Autodesk Inventor part; units mm, degrees
ref_plane "YZ Plane" through (0, 0, 0) normal (1, 0, 0) x (0, 1, 0)
ref_plane "XZ Plane" through (0, 0, 0) normal (0, 1, 0) x (-1, 0, 0)
ref_plane "XY Plane" through (0, 0, 0) normal (0, 0, 1) x (1, 0, 0)
sketch "Sketch1" plane through (0, 0, 0) normal (0, 1, 0) x (-1, 0, 0)
  circle A0 centre (0, 0) radius 73.025
  circle A1 centre (0, 0) radius 85.725
  line L0 (0, 0) -> (101.6, 0) construction
  line L1 (101.6, 0) -> (85.679, -2.8073)
  arc A2 (72.3305, -46.0117) -> (101.6, 0) centre (50.8, 0) ccw
  line L2 (-50.8, 87.9882) -> (-40.4083, 75.6039)
  arc A3 (3.6821, 85.6459) -> (-50.8, 87.9882) centre (-25.4, 43.9941) ccw
  line L3 (-50.8, -87.9882) -> (-45.2707, -72.7966)
  arc A4 (-76.0126, -39.6342) -> (-50.8, -87.9882) centre (-25.4, -43.9941) ccw
  arc A5 (78.2836, -34.935) -> (94.5805, -7.6857) centre (50.8, 0) ccw
  line L4 (94.5805, -7.6857) -> (85.215, -9.3371)
  line L5 (-40.6343, 85.752) -> (-34.5213, 78.4669)
  arc A6 (-8.8872, 85.2631) -> (-40.6343, 85.752) centre (-25.4, 43.9941) ccw
  line L6 (-53.9463, -78.0663) -> (-50.6936, -69.1298)
  arc A7 (-69.3964, -50.3281) -> (-53.9463, -78.0663) centre (-25.4, -43.9941) ccw
  point P0 (85.725, 0)
  point P1 (-42.8625, 74.24)
  point P2 (-42.8625, -74.24)
  point P3 (-8.8872, 85.2631)
  dimension "Ring_ID" = 146.05
  dimension "RingWD" = 12.7
  dimension "ToothDepth" = 15.875
  dimension "d4" = 10
  dimension "d5" = 50.8
  dimension "d8" = 360
  dimension "d13" = 6.35
  dimension "d14" = 6.35
  dimension "d17" = 360
extrude "Extrusion1" add sketch "Sketch1" along normal blind 9.525 contours A1 | A1 A6 L5 L2 A3 | L1 A2 A1 A5 L4 | A1 A7 L6 L3 A4
fillet "Fillet1" radius 3.175 6 edges at (40.4083, 4.7625, 75.6039) (-3.6821, 4.7625, 85.6459) (76.0126, 4.7625, -39.6342) (45.2707, 4.7625, -72.7966) (-85.679, 4.7625, -2.8073) (-72.3305, 4.7625, -46.0117)
fillet "Fillet2" radius 3.175 9 edges at (53.9463, 4.7625, -78.0663) (50.6936, 4.7625, -69.1298) (69.3964, 4.7625, -50.3281) (-94.5805, 4.7625, -7.6857) (-85.215, 4.7625, -9.3371) (-78.2836, 4.7625, -34.935) (40.6343, 4.7625, 85.752) (34.5213, 4.7625, 78.4669) (8.8872, 4.7625, 85.2631)
properties part number "Blade V2" material "Stainless Steel"
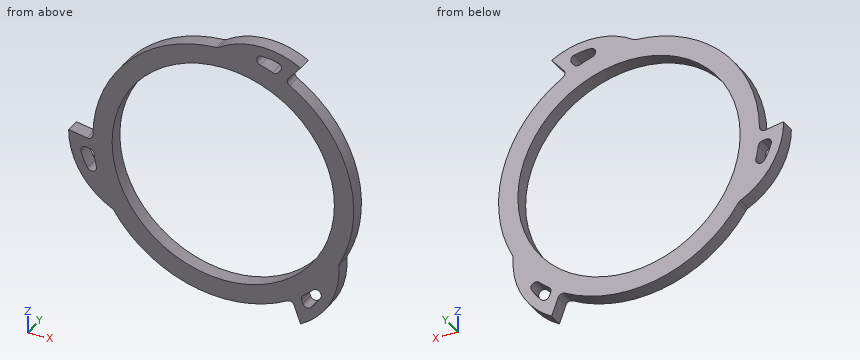
For this review, take the finished solid that the model builds, in its own axes (mm). Round coordinates to 2 decimals unless told otherwise and drop trailing zeros. Loops run counter-clockwise (first coordinate to the right, second up) from the corner with the lowest first, then second, coordinate; pieces in that order, holes last. Notation, with made-up numbers: (-34.75, 69) - (5.25, 69) arc R13 cw to (5.25, 93) - close; hole circle Ø1 at (-38, 25). An arc over 180 degrees is marked (long way). Answer as CSV lines item,"result".
(1) Consider section A-A on x = 0. Give the boundary of the cut face in (y, z) (3 decimals), then the cut area to 3 significant figures.
Checked values:
outline,"(0, -85.725) - (9.525, -85.725) - (9.525, -73.025) - (0, -73.025) - close; (0, 73.025) - (9.525, 73.025) - (9.525, 87.988) - (0, 87.988) - close"
area,"263 mm2"
(2) Consider section C-C on y = 1.5. Give the number of separate pieces and of enclosed holes in the cut face, then the cut area to 3 significant figures.
Checked values:
separate pieces,"1"
enclosed holes,"4"
area,"7,590 mm2"
(3) Wall thickness on line 1 (Z direction, x = 0, y = 3.75) (3 decimals); line 2 (Z direction, x = 35, y = 3.5); line 3 (Z direction, x = 56, y = 4.75): over which ranges is each line inside the solid? List them lowest first.
Checked values:
line 1,"z = -85.725 to -73.025, 73.025 to 87.988"
line 2,"z = -78.25 to -64.09, 64.09 to 79.46, 87.4 to 93.88"
line 3,"z = -84.54 to -75.56, -64.91 to -46.87, 46.87 to 64.91"
(4) Consider section B-B on z = 25. Give the boundary of the cut face in (x, y) (3 decimals).
Checked values:
outline,"(-81.999, 0) - (-68.612, 0) - (-68.612, 9.525) - (-81.999, 9.525) - close; (68.612, 0) - (81.999, 0) - (81.999, 9.525) - (68.612, 9.525) - close"
(5) Insertion check: P1, Ø2, axis at x = 50, y = 6.5, coming from the +Z side; P2, Ø1.5, axis at x = -15.5, y = 8, coming from the -Z side; P3, Ø5, axis at y = 2, z = -20.5, coming from the +X side. Each pin has a flat end and moves straight along its axis. Give the tip position at first contact, or say it passes through.
Checked values:
P1,"stops at z = 88.98"
P2,"stops at z = -84.45"
P3,"stops at x = 83.81"
